Study the drawing (mm; zero at the part's minimum x, y, z) and answer. A direction names the side the tool comes from. Round coordinates to 2 decimals unless told otherwise and drop trailing zeros. Loops run counter-clockwise (first coordinate to the right, second up) from the corner with the lowest first, then second, coordinate; pieces in that order, holes last. Notation, with made-up numbers: (12.25, 88.5) -> (53.25, 88.5) arc R10 ccw to (53.25, 96.5) -> close; hole circle Ø4 at (84.25, 5.25). An arc over 180 degrees is marked (long way). Use one line per item in the form item = value.
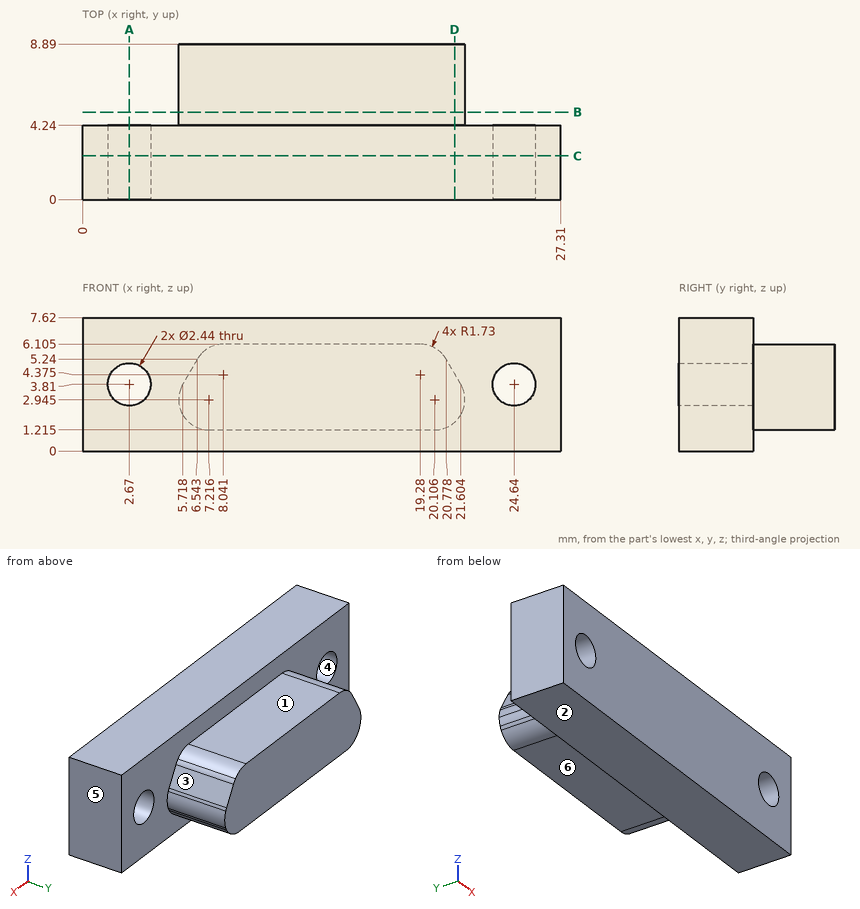
(1) For the marked faces 1, 2 and 3, determine the directions among +Z, -Z, +X, -X, +Y, -Y from which every point of the face is accessible in a straight line to the end or side of a thin tool.
Completed:
face_1 = +Z, +X, -X, +Y
face_2 = -Z, +X, -X, +Y, -Y
face_3 = +Z, +X, +Y
(2) Find section C-C, the plane y = 2.5. Write down the section's boundary in (x, z), then the cut area to 3 significant figures.
Completed:
outline = (0, 0) -> (27.31, 0) -> (27.31, 7.62) -> (0, 7.62) -> close; hole circle Ø2.44 at (2.67, 3.81); hole circle Ø2.44 at (24.64, 3.81)
area = 199 mm2
(3) Find section A-A, the plane x = 2.67. Write down the section's boundary in (y, z).
Completed:
outline = (0, 0) -> (4.24, 0) -> (4.24, 2.59) -> (0, 2.59) -> close; (0, 5.03) -> (4.24, 5.03) -> (4.24, 7.62) -> (0, 7.62) -> close
(4) Consider L1, parallel to X at y = 2.95, z = 3.81; L2, parallel to X at y = 1.25, z = 2.75 (1 decimal); L3, parallel to Y at x = 22.25, z = 3.5. Determine where each line is inside the solid, lowest interval first.
Completed:
L1 = 0 to 1.45, 3.89 to 23.42, 25.86 to 27.31
L2 = 0 to 2.1, 3.3 to 24, 25.2 to 27.3
L3 = 0 to 4.24
(5) Given P1, Ø1, axis at x = 19.5, y = 7.5, coming from the +Z side (1 decimal); P2, Ø2.5, axis at x = 15.5, y = 6, coming from the -Z side (1 decimal); P3, Ø2, axis at x = 2.67, z = 3.81, coming from the -Y side, each flat-ended and moving along its own axis, determine where each tip first touches the part or whether it passes through.
Completed:
P1 = 6.1
P2 = 1.2
P3 = through
(6) Find section B-B, the plane y = 5. Write down the section's boundary in (x, z) (1 decimal).
Completed:
outline = (5.7, 3.8) arc R1.7 ccw to (7.2, 1.2) -> (20.1, 1.2) arc R1.7 ccw to (21.6, 3.8) -> (20.8, 5.2) arc R1.7 ccw to (19.3, 6.1) -> (8, 6.1) arc R1.7 ccw to (6.5, 5.2) -> close
(7) Find section D-D, the plane x = 21.25. Write down the section's boundary in (y, z).
Completed:
outline = (0, 0) -> (4.24, 0) -> (4.24, 1.65) -> (8.89, 1.65) -> (8.89, 4.42) -> (4.24, 4.42) -> (4.24, 7.62) -> (0, 7.62) -> close
(8) For a pull along Z with two mould halves and no side action, classify the marked faces 4, 5 and 6 as +Z half, -Z half, draft (parallel to the pull), parting line (faces both ways), or undercut.
Completed:
face_4 = undercut
face_5 = draft
face_6 = -Z half
